Geometry: final body of the model. Coordinates: model frame, mm. Give positions to 0.01 mm unless a question says otherwise; leave off trailing zeros. Loops run counter-clockwise (first coordinate to the right, second up) from the corner with the lowest first, then second, coordinate; pieces in that order, holes last.
1. Section A-A, the plane y = 24.5. Output: boundary loops of the cut face in (x, z) (3 decimals), then the cut area to 3 significant figures.
2. Section C-C, the plane x = -18. Output: boundary loops of the cut face in (y, z), then the cut area to 3 significant figures.
3. Section B-B, the plane z = 53. Output: boundary loops of the cut face in (x, y), then the cut area to 3 significant figures.
4. Section D-D, the plane y = 213. Output: boundary loops of the cut face in (x, z) (3 decimals), then the cut area to 3 significant figures.
5. Material intervals for line 1 along Y through (x, z) = (-69, 24.5); line 2 along X through (y, z) = (155, 67.5); line 3 along X through (y, z) = (130, 11), sorted ascending.
6. First-contact query: P1, Ø4.5, axis at x = 59.5, y = 50, coming from the +Z side; P2, Ø3, axis at y = 185.42, z = 0, coming from the -X side (3 decimals); P3, Ø8, axis at x = -40, y = 204.5, coming from the -Z side; P4, Ø6, axis at y = 219, z = -45.5, coming from the -X side. Flat tips, straight axial feed; report the tip coordinate or a pass-through.
from build123d import *

# Parameters (mm, degrees)
SKETCH1_R           = 76.2
SKETCH1_R_2         = 73.025
BOSS_EXTRUDE1_DEPTH = 330.2
SKETCH6_W           = 88.9
SKETCH6_H           = 114.3
CUT_EXTRUDE6_DEPTH  = 20.574
CIRPATTERN9_COUNT   = 4
SKETCH7_R           = 1.7526
CUT_EXTRUDE7_DEPTH  = 17.78
CIRPATTERN10_COUNT  = 4
BOSS_EXTRUDE2_START = 25.4
SKETCH8_R           = 76.2
SKETCH8_R_2         = 73.025
BOSS_EXTRUDE2_DEPTH = 25.4


with BuildPart() as part:
    # Sketch1 → Boss-Extrude1 (new body)
    with BuildSketch(Plane(origin=(0, 0, 0), x_dir=(1, 0, 0), z_dir=(0, 1, 0))):
        with Locations(Location((0, 0, 0), (0, 0, 270))):
            Circle(SKETCH1_R)
        with Locations(Location((0, 0, 0), (0, 0, 270))):
            Circle(SKETCH1_R_2, mode=Mode.SUBTRACT)
    extrude(amount=BOSS_EXTRUDE1_DEPTH)

    # Sketch6 → Cut-Extrude6 (cut)
    with BuildSketch(Plane(origin=(0, 0, -76.2), x_dir=(-1, 0, 0), z_dir=(0, 0, -1))):
        with Locations((0, 69.85)):
            Rectangle(SKETCH6_W, SKETCH6_H)
    cut_extrude6 = extrude(amount=-CUT_EXTRUDE6_DEPTH, mode=Mode.SUBTRACT)

    # CirPattern9: Cut-Extrude6 ×4 about axis
    cirpattern9_axis = Axis((0, 0, 0), (0, 1, 0))
    for i in range(1, CIRPATTERN9_COUNT):
        add(cut_extrude6.rotate(cirpattern9_axis, i * 360 / CIRPATTERN9_COUNT), mode=Mode.SUBTRACT)

    # Sketch7 → Cut-Extrude7 (cut)
    with BuildSketch(Plane(origin=(0, 0, -76.2), x_dir=(-1, 0, 0), z_dir=(0, 0, -1))):
        with Locations(Location((0, 185.42, 0), (0, 0, 90))):
            Circle(SKETCH7_R)
        with Locations((5.55625, 144.145)):
            Circle(SKETCH7_R)
        with Locations((-5.55625, 134.62)):
            Circle(SKETCH7_R)
    cut_extrude7 = extrude(amount=-CUT_EXTRUDE7_DEPTH, mode=Mode.SUBTRACT)

    # CirPattern10: Cut-Extrude7 ×4 about axis
    cirpattern10_axis = Axis((0, 330.2, 0), (0, 1, 0))
    for i in range(1, CIRPATTERN10_COUNT):
        add(cut_extrude7.rotate(cirpattern10_axis, i * 360 / CIRPATTERN10_COUNT), mode=Mode.SUBTRACT)

    # Sketch8 → Boss-Extrude2 (add)
    with BuildSketch(Plane.XZ.offset(BOSS_EXTRUDE2_START)):
        with Locations(Location((0, 0, 0), (0, 0, 270))):
            Circle(SKETCH8_R)
        with Locations(Location((0, 0, 0), (0, 0, 270))):
            Circle(SKETCH8_R_2, mode=Mode.SUBTRACT)
    extrude(amount=-BOSS_EXTRUDE2_DEPTH)


solid = part.part
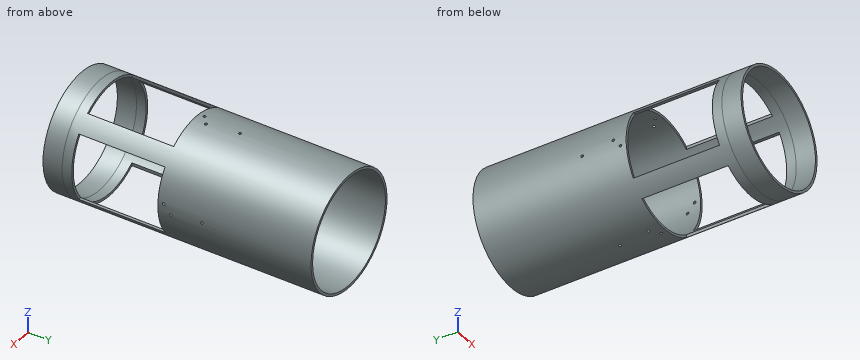
Answers below:
1. outline: (-61.892, -44.45) arc R76.2 ccw to (-44.45, -61.892) - (-44.45, -57.938) arc R73.025 cw to (-57.938, -44.45) - close; (-61.892, 44.45) - (-57.938, 44.45) arc R73.025 cw to (-44.45, 57.938) - (-44.45, 61.892) arc R76.2 ccw to start; (44.45, -61.892) arc R76.2 ccw to (61.892, -44.45) - (57.938, -44.45) arc R73.025 cw to (44.45, -57.938) - close; (44.45, 57.938) arc R73.025 cw to (57.938, 44.45) - (61.892, 44.45) arc R76.2 ccw to (44.45, 61.892) - close
1. area: 279 mm2
2. outline: (-25.4, -74.04) - (12.7, -74.04) - (12.7, -70.77) - (-25.4, -70.77) - close; (-25.4, 70.77) - (12.7, 70.77) - (12.7, 74.04) - (-25.4, 74.04) - close; (127, -74.04) - (330.2, -74.04) - (330.2, -70.77) - (127, -70.77) - close; (127, 70.77) - (330.2, 70.77) - (330.2, 74.04) - (127, 74.04) - close
2. area: 1,580 mm2
3. outline: (-54.75, -25.4) - (-50.24, -25.4) - (-50.24, 330.2) - (-54.75, 330.2) - close; (50.24, -25.4) - (54.75, -25.4) - (54.75, 330.2) - (50.24, 330.2) - close
3. area: 3,210 mm2
4. outline: circle Ø152.4 at (0, 0); hole circle Ø146.05 at (0, 0)
4. area: 1,490 mm2
5. line 1: y = -25.4 to 12.7, 127 to 330.2
5. line 2: x = -35.36 to -27.86, 27.86 to 35.36
5. line 3: x = -75.4 to -72.19, 72.19 to 75.4
6. P1: stops at z = 50.29
6. P2: passes through
6. P3: stops at z = -67.16
6. P4: stops at x = -63.25
